from build123d import *

# Parameters (mm, degrees)
F0_R     = 25.4
F1_DEPTH = 6.35
F3_D     = 6.7564
F3_DEPTH = 11.9126
F3_TIP   = 2.0298273432


with BuildPart() as f1:
    # F0 (on Front) → F1 (new body)
    with BuildSketch(Plane.XZ):
        Circle(F0_R)
        with BuildLine():
            ThreePointArc((2.5134499214, -22.7214033346), (-0.0267137561, -22.8599843914), (-2.56654661, -22.7154669443))
            Line((-2.56654661, -22.7154669443), (-2.56654661, -12.4379595794))
            ThreePointArc((-2.56654661, -12.4379595794), (-0.0270957922, -12.6999710952), (2.5134499214, -12.4487979135))
            Line((2.5134499214, -12.4487979135), (2.5134499214, -22.7214033346))
        make_face(mode=Mode.SUBTRACT)
        with BuildLine():
            ThreePointArc((-14.2891808923, -17.8437358596), (-16.1833394591, -16.1455605029), (-17.8770832263, -14.247438202))
            Line((-17.8770832263, -14.247438202), (-10.6097880749, -6.9801430506))
            ThreePointArc((-10.6097880749, -6.9801430506), (-8.9993953007, -8.9610760639), (-7.0253519387, -10.5799069059))
            Line((-7.0253519387, -10.5799069059), (-14.2891808923, -17.8437358596))
        make_face(mode=Mode.SUBTRACT)
        with BuildLine():
            ThreePointArc((17.8437358596, -14.2891808923), (16.1455605029, -16.1833394591), (14.247438202, -17.8770832263))
            Line((14.247438202, -17.8770832263), (6.9801430506, -10.6097880749))
            ThreePointArc((6.9801430506, -10.6097880749), (8.9610760639, -8.9993953007), (10.5799069059, -7.0253519387))
            Line((10.5799069059, -7.0253519387), (17.8437358596, -14.2891808923))
        make_face(mode=Mode.SUBTRACT)
        with BuildLine():
            ThreePointArc((22.7214033346, 2.5134499214), (22.8599843914, -0.0267137561), (22.7154669443, -2.56654661))
            Line((22.7154669443, -2.56654661), (12.4379595794, -2.56654661))
            ThreePointArc((12.4379595794, -2.56654661), (12.6999710952, -0.0270957922), (12.4487979135, 2.5134499214))
            Line((12.4487979135, 2.5134499214), (22.7214033346, 2.5134499214))
        make_face(mode=Mode.SUBTRACT)
        with BuildLine():
            ThreePointArc((-22.7214033346, -2.5134499214), (-22.8599843914, 0.0267137561), (-22.7154669443, 2.56654661))
            Line((-22.7154669443, 2.56654661), (-12.4379595794, 2.56654661))
            ThreePointArc((-12.4379595794, 2.56654661), (-12.6999710952, 0.0270957922), (-12.4487979135, -2.5134499214))
            Line((-12.4487979135, -2.5134499214), (-22.7214033346, -2.5134499214))
        make_face(mode=Mode.SUBTRACT)
        with BuildLine():
            ThreePointArc((-17.8437358596, 14.2891808923), (-16.1455605029, 16.1833394591), (-14.247438202, 17.8770832263))
            Line((-14.247438202, 17.8770832263), (-6.9801430506, 10.6097880749))
            ThreePointArc((-6.9801430506, 10.6097880749), (-8.9610760639, 8.9993953007), (-10.5799069059, 7.0253519387))
            Line((-10.5799069059, 7.0253519387), (-17.8437358596, 14.2891808923))
        make_face(mode=Mode.SUBTRACT)
        with BuildLine():
            ThreePointArc((14.2891808923, 17.8437358596), (16.1833394591, 16.1455605029), (17.8770832263, 14.247438202))
            Line((17.8770832263, 14.247438202), (10.6097880749, 6.9801430506))
            ThreePointArc((10.6097880749, 6.9801430506), (8.9993953007, 8.9610760639), (7.0253519387, 10.5799069059))
            Line((7.0253519387, 10.5799069059), (14.2891808923, 17.8437358596))
        make_face(mode=Mode.SUBTRACT)
        with BuildLine():
            Line((-2.5134499214, 12.4487979135), (-2.5134499214, 22.7214033346))
            ThreePointArc((-2.5134499214, 22.7214033346), (0.0267137561, 22.8599843914), (2.56654661, 22.7154669443))
            Line((2.56654661, 22.7154669443), (2.56654661, 12.4379595794))
            ThreePointArc((2.56654661, 12.4379595794), (0.0270957922, 12.6999710952), (-2.5134499214, 12.4487979135))
        make_face(mode=Mode.SUBTRACT)
    extrude(amount=F1_DEPTH)

    # F3
    with Locations(Plane.XZ.offset(6.35)):
        with Locations((0, 0)):
            Hole(F3_D / 2, depth=F3_DEPTH)
            with Locations((0, 0, -(F3_DEPTH + F3_TIP / 2))):  # 118° drill point
                Cone(0, F3_D / 2, F3_TIP, mode=Mode.SUBTRACT)


solid = f1.part
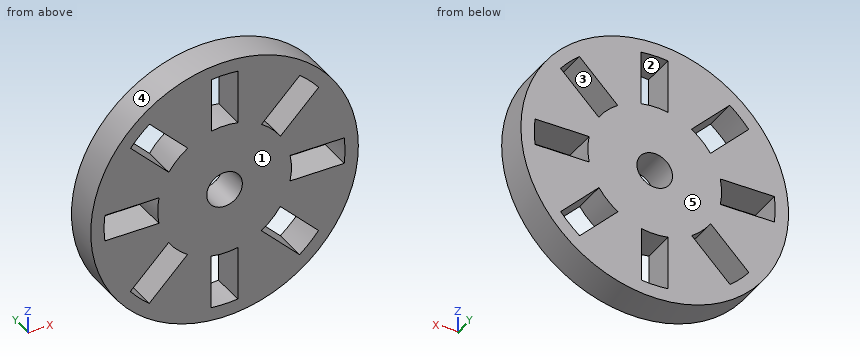
Geometry: final body of the model. Coordinates: model frame, mm. Face numbers are marked on the shaded views. A direction names the side the tool comes from. Give positions to 0.01 mm unless a question says otherwise; leave off trailing zeros. Write each loop counter-clockwise with the first axis right and the second up, starting at its lowest first coordinate (ties: lowest second). Pieces come first, ordered by that corner, then holes. Notation, with made-up numbers: (19, 12) - (30, 12) arc R12 ccw to (30, 16) - close; hole circle Ø11 at (2.5, 14). An arc over 180 degrees is marked (long way). Return JSON: item names as keys, results as strings. Group by question number.
1) Section A-A on x = 0. Return the cut outline in (y, z).
2) Line query: line 1 (Z direction, x = 0, y = -4.5); line 2 (X direction, y = -3.25, z = 13.5); line 3 (X direction, y = -0.25, z = -11.5). Output: solid intervals per line, ascending.
3) Section D-D on y = -2. State how many separate pieces and enclosed holes the cut face has, plus the area to 3 significant figures.
4) Mould query, pull axis X, two halves, no side actions, for the marked faces 3, 4 and 5. Classes: released by +X, released by -X, zero draft, split by the parting line, or undercut.
5) First-contact query: P1, Ø3, axis at x = 17, y = -3, coming from the +Z side; P2, Ø1.9, axis at x = -15.5, y = -3.5, coming from the +Z side; P3, Ø3, axis at x = -2, z = 1.5, coming from the -Y side; P4, Ø3, axis at y = -3, z = 17, coming from the +X side. Flat tips, straight axial feed; report the tip coordinate or a pass-through.
6) Set-up query: the marked faces 1 and 2. Return all of +Z, -Z, +X, -X, +Y, -Y with unobstructed straight access to the full face (end or side cutting, diameter ignored); none if empty.
7) Section B-B on z = 0. Return the cut outline in (x, y).
8) Section C-C on x = 9.5. Return the cut outline in (y, z).
Filled in:
{
 "1": {"outline": "(-6.35, -25.4) - (0, -25.4) - (0, -22.86) - (-6.35, -22.86) - close; (-6.35, -12.7) - (0, -12.7) - (0, -3.38) - (-6.35, -3.38) - close; (-6.35, 3.38) - (0, 3.38) - (0, 12.7) - (-6.35, 12.7) - close; (-6.35, 22.86) - (0, 22.86) - (0, 25.4) - (-6.35, 25.4) - close"},
 "2": {"line 1": "z = -25.4 to -22.86, -12.7 to -3.38, 3.38 to 12.7, 22.86 to 25.4", "line 2": "x = -21.52 to -17.05, -9.87 to -2.51, 2.57 to 9.95, 17.13 to 21.52", "line 3": "x = -22.65 to -15.13, -7.95 to 7.87, 15.05 to 22.65"},
 "3": {"separate pieces": "1", "enclosed holes": "9", "area": "1,580 mm^2"},
 "4": {"face 3": "undercut", "face 4": "split by the parting line", "face 5": "zero draft"},
 "5": {"P1": "stops at z = 20.12", "P2": "stops at z = 20.82", "P3": "stops at y = -6.35", "P4": "stops at x = 20.12"},
 "6": {"face 1": "+Z, -Z, +X, -X, -Y", "face 2": "+Y, -Y"},
 "7": {"outline": "(-25.4, -6.35) - (-22.86, -6.35) - (-22.86, 0) - (-25.4, 0) - close; (-12.7, -6.35) - (-3.38, -6.35) - (-3.38, 0) - (-12.7, 0) - close; (3.38, -6.35) - (12.7, -6.35) - (12.7, 0) - (3.38, 0) - close; (22.86, -6.35) - (25.4, -6.35) - (25.4, 0) - (22.86, 0) - close"},
 "8": {"outline": "(-6.35, -23.56) - (0, -23.56) - (0, -13.13) - (-6.35, -13.13) - close; (-6.35, -8.43) - (0, -8.43) - (0, 8.43) - (-6.35, 8.43) - close; (-6.35, 13.05) - (0, 13.05) - (0, 23.56) - (-6.35, 23.56) - close"}
}
